Geometry check sheet. Reference: the model listing, model coordinates, mm. Face numbers are marked on the shaded views. Coordinates: 2 decimals unless noted, no trailing zeros. Order: outer loops, then holes, each group sorted by start corner. A loop starts at its lowest first (then second) coordinate and runs counter-clockwise, first axis right, second up. Notation, with made-up numbers: (27, 13.25) - (69, 13.25) arc R8 ccw to (69, 18.25) - close; hole circle Ø8 at (40.25, 65.5). An arc over 180 degrees is marked (long way). Use CSV: the item, a comma, the result in double quotes. Start each with the question number.
1) Sectioned sample at B-B, the plane x = -0.5. Record the cut outline in (y, z), and give its area (3 significant figures).
2) Sectioned sample at D-D, the plane z = 30. Record the cut outline in (x, y), and give its area (3 significant figures).
3) Thickness scan on probe 1 along X at (y, z) = (12.5, 8.5); probe 2 along Y at (x, z) = (-0.5, 19.5); probe 3 along Y at (x, z) = (-16, 29.5). Record the ranges inside material, lowest first. Write a range as [from, to].
4) Depth check by flat-ended pin: P1, Ø1.2, axis at x = 18, z = 30, coming from the +Y side; P2, Ø12, axis at x = -18.5, y = -8.5, coming from the -Z side; P3, Ø4, axis at x = -16, y = 0, coming from the +Z side. Enter the tip coordinate at first touch or a pass-through.
5) Sectioned sample at C-C, the plane x = -13. Record the cut outline in (y, z).
6) Sectioned sample at A-A, the plane y = 0. Record the cut outline in (x, z).
7) Draft check along Y on the marked faces 1, 2 and 3. Enter one of: released by +Y, released by -Y, zero draft, split by the parting line, or undercut.
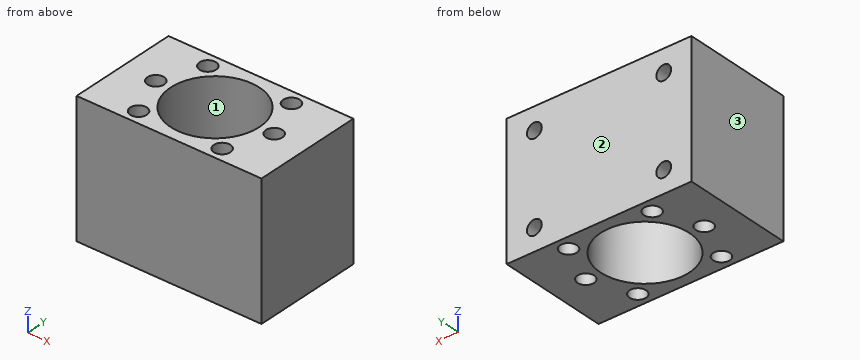
from build123d import *

# Parameters (mm, degrees)
SKETCH_1_W          = 50
SKETCH_1_H          = 30
SKETCH_1_R          = 2.25
SKETCH_1_R_2        = 12
EXTRUDE_1_DEPTH     = 36
SKETCH_2_R          = 2
CUT_EXTRUDE_1_DEPTH = 10.2


with BuildPart() as part:
    # 草图1 → 凸台-拉伸1 (new body)
    with BuildSketch(Plane.XY):
        Rectangle(SKETCH_1_W, SKETCH_1_H)
        with Locations((-11.313708499, 11.313708499)):
            Circle(SKETCH_1_R, mode=Mode.SUBTRACT)
        with Locations((-16, 0)):
            Circle(SKETCH_1_R, mode=Mode.SUBTRACT)
        with Locations((-11.313708499, -11.313708499)):
            Circle(SKETCH_1_R, mode=Mode.SUBTRACT)
        with Locations((11.313708499, -11.313708499)):
            Circle(SKETCH_1_R, mode=Mode.SUBTRACT)
        with Locations((16, 0)):
            Circle(SKETCH_1_R, mode=Mode.SUBTRACT)
        with Locations((11.313708499, 11.313708499)):
            Circle(SKETCH_1_R, mode=Mode.SUBTRACT)
        Circle(SKETCH_1_R_2, mode=Mode.SUBTRACT)
    extrude(amount=EXTRUDE_1_DEPTH)

    # 草图2 → 切除-拉伸1 (cut)
    with BuildSketch(Plane(origin=(0, 15, 0), x_dir=(1, 0, 0), z_dir=(0, 1, 0))):
        with Locations(Location((17.5, -30, 0), (0, 0, 270))):
            Circle(SKETCH_2_R)
        with Locations(Location((-17.5, -30, 0), (0, 0, 90))):
            Circle(SKETCH_2_R)
        with Locations(Location((-17.5, -6, 0), (0, 0, 270))):
            Circle(SKETCH_2_R)
        with Locations(Location((17.5, -6, 0), (0, 0, 90))):
            Circle(SKETCH_2_R)
    extrude(amount=-CUT_EXTRUDE_1_DEPTH, mode=Mode.SUBTRACT)


solid = part.part
Evaluation:
1,outline,"(-15, 0) - (-11.99, 0) - (-11.99, 36) - (-15, 36) - close; (11.99, 0) - (15, 0) - (15, 36) - (11.99, 36) - close"
1,area,"217 mm²"
2,outline,"(-25, -15) - (25, -15) - (25, 15) - (19.5, 15) - (19.5, 4.8) - (15.5, 4.8) - (15.5, 15) - (-15.5, 15) - (-15.5, 4.8) - (-19.5, 4.8) - (-19.5, 15) - (-25, 15) - close; hole circle Ø4.5 at (-16, 0); hole circle Ø4.5 at (-11.31, -11.31); hole circle Ø4.5 at (-11.31, 11.31); hole circle Ø24 at (0, 0); hole circle Ø4.5 at (11.31, -11.31); hole circle Ø4.5 at (11.31, 11.31); hole circle Ø4.5 at (16, 0)"
2,area,"871 mm²"
3,probe 1,"[-25, -13.23], [-9.4, 9.4], [13.23, 25]"
3,probe 2,"[-15, -11.99], [11.99, 15]"
3,probe 3,"[-15, -2.25], [2.25, 4.8]"
4,P1,"y = 4.8"
4,P2,"z = 0"
4,P3,"through"
5,outline,"(-15, 0) - (-12.8, 0) - (-12.8, 36) - (-15, 36) - close; (-9.82, 0) - (9.82, 0) - (9.82, 36) - (-9.82, 36) - close; (12.8, 0) - (15, 0) - (15, 36) - (12.8, 36) - close"
6,outline,"(-25, 0) - (-18.25, 0) - (-18.25, 36) - (-25, 36) - close; (-13.75, 0) - (-12, 0) - (-12, 36) - (-13.75, 36) - close; (12, 0) - (13.75, 0) - (13.75, 36) - (12, 36) - close; (18.25, 0) - (25, 0) - (25, 36) - (18.25, 36) - close"
7,face 1,"undercut"
7,face 2,"released by +Y"
7,face 3,"zero draft"
